Input: dimensioned drawing with shaded views. Units: mm. Origin: part minimum x, y, z. Coordinates: 2 decimals unless noted, no trailing zeros. Loops run counter-clockwise (first coordinate to the right, second up) from the corner with the lowest first, then second, coordinate; pieces in that order, holes last. Notation, with made-up numbers: (72, -19.5) - (95, -19.5) arc R30 ccw to (95, 2.5) - close; hole circle Ø9 at (53, 87.5). An arc over 180 degrees is marked (long way). Put each result on its own line as item: value. Start each with the question number.
1) Material intervals for line 1 along Z through (x, y) = (80.5, 10.5); line 2 along Z through (x, y) = (6.35, 7.25); line 3 along X through (y, z) = (4, 9) (1 decimal), sorted ascending. Write a range as from..to.
2) Contact query for a flat-ended pin moving along its axis: pin 1 Ø5 at (x, z) = (19.05, 6.35) entering from -Y. Output: stop coordinate, or through.
3) Section C-C on x = 73. Output: boundary loops of the cut face in (y, z).
4) Section A-A on z = 6.35. Output: boundary loops of the cut face in (x, y) (1 decimal), and give its area (3 significant figures).
5) Section B-B on x = 19.05. Count the separate pieces of the cut face and the enclosed holes in it, and give its area (3 significant figures).
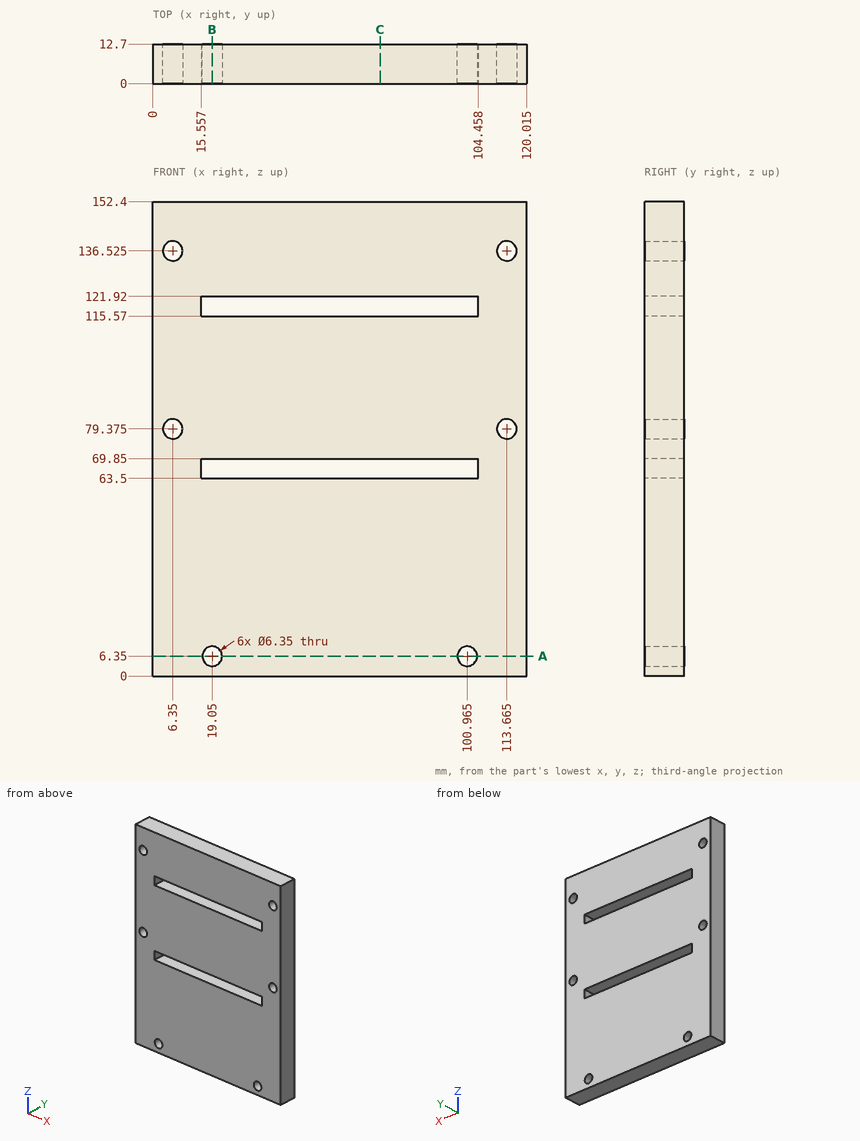
Answer block:
1. line 1: z = 0..63.5, 69.85..115.57, 121.92..152.4
1. line 2: z = 0..76.2, 82.55..133.35, 139.7..152.4
1. line 3: x = 0..17.3, 20.8..99.2, 102.7..120
2. pin 1: passes through
3. outline: (0, 0) - (12.7, 0) - (12.7, 63.5) - (0, 63.5) - close; (0, 69.85) - (12.7, 69.85) - (12.7, 115.57) - (0, 115.57) - close; (0, 121.92) - (12.7, 121.92) - (12.7, 152.4) - (0, 152.4) - close
4. outline: (0, 0) - (15.9, 0) - (15.9, 12.7) - (0, 12.7) - close; (22.2, 0) - (97.8, 0) - (97.8, 12.7) - (22.2, 12.7) - close; (104.1, 0) - (120, 0) - (120, 12.7) - (104.1, 12.7) - close
4. area: 1,360 mm²
5. separate pieces: 4
5. enclosed holes: 0
5. area: 1,690 mm²
